Autodesk Inventor part; units mm, degrees
ref_plane "Work Plane1" through (0, 0, 0) normal (0, 0, 1) x (1, 0, 0)
ref_plane "YZ Plane" through (0, 0, 0) normal (1, 0, 0) x (0, 1, 0)
ref_plane "XZ Plane" through (0, 0, 0) normal (0, 1, 0) x (-1, 0, 0)
ref_plane "Work Plane1" through (0, 0, 0) normal (0, 0, 1) x (1, 0, 0)
sketch "Sketch1" plane through (0, 0, 0) normal (0, 0, 1) x (1, 0, 0)
  circle A0 centre (0, 0) radius 21
  circle A1 centre (23.57, -23.57) radius 2
  circle A2 centre (23.57, 23.57) radius 2
  circle A3 centre (-23.57, -23.57) radius 2.5
  circle A4 centre (-23.57, 23.57) radius 2
  circle A5 centre (-23.57, -23.57) radius 2
  circle A6 centre (0, 0) radius 19
  circle A7 centre (-23.57, 23.57) radius 2.5
  circle A8 centre (-23.57, -23.57) radius 2.5
  arc A9 (-29.95, -24.95) -> (-24.95, -29.95) centre (-24.95, -24.95) ccw
  line L0 (24.95, -29.95) -> (-24.95, -29.95)
  arc A10 (24.95, -29.95) -> (29.95, -24.95) centre (24.95, -24.95) ccw
  line L1 (29.95, 24.95) -> (29.95, -24.95)
  arc A11 (29.95, 24.95) -> (24.95, 29.95) centre (24.95, 24.95) ccw
  line L2 (-24.95, 29.95) -> (24.95, 29.95)
  arc A12 (-24.95, 29.95) -> (-29.95, 24.95) centre (-24.95, 24.95) ccw
  line L3 (-29.95, -24.95) -> (-29.95, 24.95)
  circle A13 centre (23.57, -23.57) radius 2.5
  circle A14 centre (23.57, 23.57) radius 2.5
  line L4 (-49.95, -90) -> (-49.95, 90)
  line L5 (-59.95, -90) -> (-49.95, -90)
  line L6 (-59.95, 90) -> (-49.95, 90)
  line L7 (40.2846, 0) -> (-40.2846, 0)
  line L8 (-49.95, -90) -> (-49.95, 90)
  line L9 (-59.95, -90) -> (-49.95, -90)
  line L10 (-49.95, 35.5095) -> (-26.95, 35.5095)
  line L11 (-24.95, 29.95) -> (-49.95, 29.95)
  line L12 (-24.95, -29.95) -> (-49.95, -29.95)
  circle A15 centre (0, 0) radius 22
  line L13 (-32.95, 22) -> (-32.95, -22)
  line L14 (-30.95, -14.95) -> (-49.95, -14.95)
  line L15 (-30.95, 14.95) -> (-49.95, 14.95)
  line L16 (-30.95, -14.95) -> (-30.95, 14.95)
  line L17 (24.7214, -34.026) -> (0, -42.0585)
  line L18 (0, -42.0585) -> (-24.7214, -34.026)
  line L19 (-24.7214, -34.026) -> (-40, -12.9968)
  line L20 (-40, -12.9968) -> (-40, 12.9968)
  line L21 (-40, 12.9968) -> (-24.7214, 34.026)
  line L22 (-24.7214, 34.026) -> (0, 42.0585)
  line L23 (0, 42.0585) -> (24.7214, 34.026)
  line L24 (24.7214, 34.026) -> (40, 12.9968)
  line L25 (40, 12.9968) -> (40, -12.9968)
  line L26 (40, -12.9968) -> (24.7214, -34.026)
  line L27 (-24.7214, -34.026) -> (-49.95, -34.026)
  line L28 (-24.7214, 34.026) -> (-49.95, 34.026)
  arc A16 (-24.7214, -34.026) -> (-24.7214, 34.026) centre (0, 0) ccw
  line L29 (-24.7214, 34.026) -> (-27.8, 34.026)
  line L30 (-27.8, 34.026) -> (-27.8, 80.5095)
  line L31 (-27.8, 80.5095) -> (-49.95, 80.5095)
  line L32 (-49.95, 80.5095) -> (-49.95, 14.95)
  line L33 (-49.95, 14.95) -> (-35.95, 14.95)
  arc A17 (-30.95, 9.95) -> (-35.95, 14.95) centre (-35.95, 9.95) ccw
  line L34 (-30.95, 9.95) -> (-30.95, -9.95)
  arc A18 (-35.95, -14.95) -> (-30.95, -9.95) centre (-35.95, -9.95) ccw
  line L35 (-35.95, -14.95) -> (-49.95, -14.95)
  line L36 (-49.95, -14.95) -> (-49.95, -34.026)
  line L37 (-49.95, -34.026) -> (-24.7214, -34.026)
  circle A19 centre (15.9909, -0.539) radius 1.6
  circle A20 centre (-11.6884, -10.9261) radius 2
  circle A21 centre (11.6884, 10.9261) radius 2
  circle A22 centre (10.9261, -11.6884) radius 2
  circle A23 centre (-15.9909, 0.539) radius 1.6
  circle A24 centre (-0.539, -15.9909) radius 1.6
  circle A25 centre (0, 0) radius 12.5
  circle A26 centre (0.539, 15.9909) radius 1.6
  circle A27 centre (-10.9261, 11.6884) radius 2
  point P0 (0, 0)
  point P1 (-23.2856, -45.1645)
  point P2 (-49.95, -75.9684)
  point P3 (-23.2856, 45.1645)
  point P4 (-49.95, -14.95)
  point P5 (-32.95, 13.95)
  point P6 (-32.95, 14.95)
  dimension "d9" = 1
  dimension "d10" = 15
  dimension "d11" = 15
  dimension "d12" = 1
  dimension "d13" = 40
extrude "Extrusion1" add sketch "Sketch1" along normal blind 10 contours L7 A15 A0 | A0 L7 A15 | A15 L7 L3 A12 L2 A11 L1 | L7 L1 A10 L0 A9 L3 A15 | L7 L25 L26 L17 L18 L19 L12 L0 A10 L1 | L1 A11 L2 L11 L21 L22 L23 L24 L25 L7 | L7 L16 L15 L21 L11 A12 L3 | L3 A9 L12 L19 L14 L16 L7 | L25 A16 | L16 A18 L13 L7 | L7 L13 A17 L16 | L24 A16 | A16 L26 | L13 A18 L14 L19 L20 L7 | L7 L20 L21 L15 A17 L13 | L16 L14 L13 A18 | A17 L13 L15 L16 | L23 A16 | A16 L17 | L19 L27 L4 L12 | L12 L4 L14 L19 | L21 L15 L4 L11 | L11 L4 L28 L21 | L20 L19 L14 L4 L15 L21 | A17 L15 L13 | L13 L14 A18 | L22 A16 | A16 L18 | A1 | A2 | A3 | A4 | A5 | A7 | A13 | A14
sketch "Sketch2" plane through (-49.95, -34.026, 0) normal (-1, 0, 0) x (0, 0, 1)
  line L0 (0, 68.0521) -> (0, 0)
  line L1 (0, 0) -> (10, 0)
  line L2 (10, 68.0521) -> (10, 0)
  line L3 (0, 68.0521) -> (0, 0)
  line L4 (10, 68.0521) -> (10, 0)
  line L5 (0, 68.0521) -> (10, 68.0521)
  line L6 (0, 0) -> (10, 0)
  line L7 (0, 68.0521) -> (10, 68.0521)
  point P0 (0, 34.026)
  point P1 (5, 7.5)
  point P2 (5, 60.5521)
  point P3 (5, 68.0521)
  point P4 (5, 19.076)
  dimension "d24" = 7.5
  dimension "d25" = 7.5
hole "Hole1" at (-49.95, 26.526, 5) at (-49.95, -26.526, 5) direction (1, 0, 0) diameter 3.242 depth 15 tip angle 118
sketch "Sketch3" plane through (0, 0, 10) normal (0, 0, 1) x (1, 0, 0)
  arc A0 (-24.7214, -34.026) -> (-24.7214, 34.026) centre (0, 0) ccw
  line L0 (-24.7214, 34.026) -> (-27.8, 34.026)
  line L1 (-27.8, 34.026) -> (-27.8, 80.5095)
  line L2 (-27.8, 80.5095) -> (-49.95, 80.5095)
  line L3 (-49.95, 80.5095) -> (-49.95, 14.95)
  line L4 (-49.95, 14.95) -> (-35.95, 14.95)
  arc A1 (-30.95, 9.95) -> (-35.95, 14.95) centre (-35.95, 9.95) ccw
  line L5 (-30.95, 9.95) -> (-30.95, -9.95)
  arc A2 (-35.95, -14.95) -> (-30.95, -9.95) centre (-35.95, -9.95) ccw
  line L6 (-35.95, -14.95) -> (-49.95, -14.95)
  line L7 (-49.95, -14.95) -> (-49.95, -34.026)
  line L8 (-49.95, -34.026) -> (-24.7214, -34.026)
  circle A3 centre (15.9909, -0.539) radius 1.6
  circle A4 centre (-11.6884, -10.9261) radius 2
  circle A5 centre (11.6884, 10.9261) radius 2
  circle A6 centre (10.9261, -11.6884) radius 2
  circle A7 centre (-15.9909, 0.539) radius 1.6
  circle A8 centre (-0.539, -15.9909) radius 1.6
  circle A9 centre (0, 0) radius 12.5
  circle A10 centre (0.539, 15.9909) radius 1.6
  circle A11 centre (-10.9261, 11.6884) radius 2
  circle A12 centre (0, 0) radius 19
  circle A13 centre (-23.57, 23.57) radius 2.5
  circle A14 centre (-23.57, -23.57) radius 2.5
  arc A15 (-29.95, -24.95) -> (-24.95, -29.95) centre (-24.95, -24.95) ccw
  line L9 (24.95, -29.95) -> (-24.95, -29.95)
  arc A16 (24.95, -29.95) -> (29.95, -24.95) centre (24.95, -24.95) ccw
  line L10 (29.95, 24.95) -> (29.95, -24.95)
  arc A17 (29.95, 24.95) -> (24.95, 29.95) centre (24.95, 24.95) ccw
  line L11 (-24.95, 29.95) -> (24.95, 29.95)
  arc A18 (-24.95, 29.95) -> (-29.95, 24.95) centre (-24.95, 24.95) ccw
  line L12 (-29.95, -24.95) -> (-29.95, 24.95)
  circle A19 centre (23.57, -23.57) radius 2.5
  circle A20 centre (23.57, 23.57) radius 2.5
  arc A21 (-37.4079, -14.95) -> (-37.4079, 14.95) centre (0, 0) ccw
  line L13 (-27.8, 34.026) -> (-27.8, 29.155)
  line L14 (-49.95, -34.026) -> (-21.5657, -34.026)
  line L15 (-49.95, -34.026) -> (-24.7214, -34.026)
  point P0 (0, 0)
  point P1 (-24.7214, -34.026)
extrude "Extrusion2" cut sketch "Sketch3" against normal blind 10 contours L14 A21 L13 L0 A0
sketch "Sketch4" plane through (0, 0, 10) normal (0, 0, 1) x (1, 0, 0)
  arc A0 (-24.7214, -34.026) -> (-24.7214, 34.026) centre (0, 0) ccw
  line L0 (-24.7214, 34.026) -> (-27.8, 34.026)
  line L1 (-27.8, 34.026) -> (-27.8, 80.5095)
  line L2 (-27.8, 80.5095) -> (-49.95, 80.5095)
  line L3 (-49.95, 80.5095) -> (-49.95, 14.95)
  line L4 (-49.95, 14.95) -> (-35.95, 14.95)
  arc A1 (-30.95, 9.95) -> (-35.95, 14.95) centre (-35.95, 9.95) ccw
  line L5 (-30.95, 9.95) -> (-30.95, -9.95)
  arc A2 (-35.95, -14.95) -> (-30.95, -9.95) centre (-35.95, -9.95) ccw
  line L6 (-35.95, -14.95) -> (-49.95, -14.95)
  line L7 (-49.95, -14.95) -> (-49.95, -34.026)
  line L8 (-49.95, -34.026) -> (-24.7214, -34.026)
  circle A3 centre (15.9909, -0.539) radius 1.6
  circle A4 centre (-11.6884, -10.9261) radius 2
  circle A5 centre (11.6884, 10.9261) radius 2
  circle A6 centre (10.9261, -11.6884) radius 2
  circle A7 centre (-15.9909, 0.539) radius 1.6
  circle A8 centre (-0.539, -15.9909) radius 1.6
  circle A9 centre (0, 0) radius 12.5
  circle A10 centre (0.539, 15.9909) radius 1.6
  circle A11 centre (-10.9261, 11.6884) radius 2
  line L9 (-49.95, -90) -> (-49.95, 90)
  line L10 (-59.95, 90) -> (-49.95, 90)
  line L11 (-49.95, -90) -> (-49.95, 90)
  line L12 (-27.8, 29.155) -> (-27.8, 34.026)
  line L13 (-27.8, 34.026) -> (-49.95, 34.026)
  line L14 (-49.95, 34.026) -> (-49.95, -34.026)
  line L15 (-49.95, -34.026) -> (-21.5657, -34.026)
  arc A12 (-21.5657, -34.026) -> (-27.8, 29.155) centre (0, 0) ccw
  circle A13 centre (0, 0) radius 21
  point P0 (0, 0)
extrude "Extrusion3" add sketch "Sketch4" against normal blind 10 contours L13 L3 L2 L1
fillet "Fillet1" radius 2 2 edges at (-27.8, 29.155, 5) (-21.5657, -34.026, 5)
fillet "Fillet2" radius 1 1 edges at (-27.8, 80.5095, 5)
sketch "Sketch5" plane through (-27.8, 33.5015, 10) normal (1, 0, 0) x (0, 0, -1)
  arc A0 (8, 9.19) -> (10, 11.19) centre (8, 11.19) ccw
  line L0 (10, 49.19) -> (10, 11.19)
  arc A1 (10, 49.19) -> (8, 51.19) centre (8, 49.19) ccw
  line L1 (-60.5, 51.19) -> (8, 51.19)
  arc A2 (-60.5, 51.19) -> (-62.5, 49.19) centre (-60.5, 49.19) ccw
  line L2 (-62.5, 11.19) -> (-62.5, 49.19)
  arc A3 (-62.5, 11.19) -> (-60.5, 9.19) centre (-60.5, 11.19) ccw
  line L3 (8, 9.19) -> (-60.5, 9.19)
  circle A4 centre (-26.25, 30.19) radius 12.6
  circle A5 centre (-26.25, 14.19) radius 2
  arc A6 (-59.6, 14.79) -> (-55.4, 14.79) centre (-57.5, 14.79) ccw
  line L4 (-59.6, 45.59) -> (-59.6, 14.79)
  arc A7 (-55.4, 45.59) -> (-59.6, 45.59) centre (-57.5, 45.59) ccw
  line L5 (-55.4, 14.79) -> (-55.4, 45.59)
  circle A8 centre (-42.25, 30.19) radius 2
  circle A9 centre (-37.5637, 18.8763) radius 1.5
  circle A10 centre (-37.5637, 41.5037) radius 1.5
  circle A11 centre (-14.9363, 18.8763) radius 1.5
  arc A12 (7.1, 45.59) -> (2.9, 45.59) centre (5, 45.59) ccw
  line L6 (7.1, 14.79) -> (7.1, 45.59)
  arc A13 (2.9, 14.79) -> (7.1, 14.79) centre (5, 14.79) ccw
  line L7 (2.9, 45.59) -> (2.9, 14.79)
  circle A14 centre (-10.25, 30.19) radius 2
  circle A15 centre (-14.9363, 41.5037) radius 1.5
  circle A16 centre (-26.25, 46.19) radius 2
  circle A17 centre (-57.5, 11.46) radius 1.621
  circle A18 centre (-57.5, 26.86) radius 1.621
  arc A19 (8, 9.19) -> (10, 11.19) centre (8, 11.19) ccw
  line L8 (10, 49.19) -> (10, 11.19)
  arc A20 (10, 49.19) -> (8, 51.19) centre (8, 49.19) ccw
  line L9 (-60.5, 51.19) -> (8, 51.19)
  arc A21 (-60.5, 51.19) -> (-62.5, 49.19) centre (-60.5, 49.19) ccw
  line L10 (-62.5, 11.19) -> (-62.5, 49.19)
  arc A22 (-62.5, 11.19) -> (-60.5, 9.19) centre (-60.5, 11.19) ccw
  line L11 (8, 9.19) -> (-60.5, 9.19)
  circle A23 centre (-26.25, 30.19) radius 12.6
  circle A24 centre (-26.25, 14.19) radius 2
  arc A25 (-59.6, 14.79) -> (-55.4, 14.79) centre (-57.5, 14.79) ccw
  line L12 (-59.6, 45.59) -> (-59.6, 14.79)
  arc A26 (-55.4, 45.59) -> (-59.6, 45.59) centre (-57.5, 45.59) ccw
  line L13 (-55.4, 14.79) -> (-55.4, 45.59)
  circle A27 centre (-42.25, 30.19) radius 2
  circle A28 centre (-37.5637, 18.8763) radius 1.5
  circle A29 centre (-37.5637, 41.5037) radius 1.5
  circle A30 centre (-14.9363, 18.8763) radius 1.5
  arc A31 (7.1, 45.59) -> (2.9, 45.59) centre (5, 45.59) ccw
  line L14 (7.1, 14.79) -> (7.1, 45.59)
  arc A32 (2.9, 14.79) -> (7.1, 14.79) centre (5, 14.79) ccw
  line L15 (2.9, 45.59) -> (2.9, 14.79)
  circle A33 centre (-10.25, 30.19) radius 2
  circle A34 centre (-14.9363, 41.5037) radius 1.5
  circle A35 centre (-26.25, 46.19) radius 2
  arc A36 (8, 9.19) -> (10, 11.19) centre (8, 11.19) ccw
  line L16 (10, 49.19) -> (10, 11.19)
  arc A37 (10, 49.19) -> (8, 51.19) centre (8, 49.19) ccw
  line L17 (-60.5, 51.19) -> (8, 51.19)
  arc A38 (-60.5, 51.19) -> (-62.5, 49.19) centre (-60.5, 49.19) ccw
  line L18 (-62.5, 11.19) -> (-62.5, 49.19)
  arc A39 (-62.5, 11.19) -> (-60.5, 9.19) centre (-60.5, 11.19) ccw
  line L19 (8, 9.19) -> (-60.5, 9.19)
  circle A40 centre (-26.25, 30.19) radius 12.6
  circle A41 centre (-26.25, 14.19) radius 2
  arc A42 (-59.6, 14.79) -> (-55.4, 14.79) centre (-57.5, 14.79) ccw
  line L20 (-59.6, 45.59) -> (-59.6, 14.79)
  arc A43 (-55.4, 45.59) -> (-59.6, 45.59) centre (-57.5, 45.59) ccw
  line L21 (-55.4, 14.79) -> (-55.4, 45.59)
  circle A44 centre (-42.25, 30.19) radius 2
  circle A45 centre (-37.5637, 18.8763) radius 1.5
  circle A46 centre (-37.5637, 41.5037) radius 1.5
  circle A47 centre (-14.9363, 18.8763) radius 1.5
  arc A48 (7.1, 45.59) -> (2.9, 45.59) centre (5, 45.59) ccw
  line L22 (7.1, 14.79) -> (7.1, 45.59)
  arc A49 (2.9, 14.79) -> (7.1, 14.79) centre (5, 14.79) ccw
  line L23 (2.9, 45.59) -> (2.9, 14.79)
  circle A50 centre (-10.25, 30.19) radius 2
  circle A51 centre (-14.9363, 41.5037) radius 1.5
  circle A52 centre (-26.25, 46.19) radius 2
  point P0 (10, -33.5015)
  point P1 (5, 22.29)
  point P2 (5, 38.09)
  dimension "d47" = 7.5
  dimension "d48" = 7.5
hole "Hole2" at (-27.8, 55.7915, 5) at (-27.8, 71.5915, 5) direction (-1, 0, 0) diameter 3.242 depth 22.15
sketch "Sketch7" plane through (0, 0, 10) normal (0, 0, 1) x (1, 0, 0)
  circle A0 centre (0, 0) radius 32.55
  dimension "d49" = 65.1
extrude "Extrusion5" cut sketch "Sketch7" against normal blind 7
sketch "Sketch10" plane through (0, 0, 0) normal (0, 0, -1) x (-1, 0, 0)
  point P0 (0, 0)
  point P1 (-23.57, -23.57)
  point P2 (-23.57, 23.57)
  point P3 (23.57, 23.57)
  point P4 (23.57, -23.57)
hole "Hole3" at (23.57, -23.57, 0) at (23.57, 23.57, 0) at (-23.57, 23.57, 0) at (-23.57, -23.57, 0) direction (0, 0, 1) diameter 3.242 depth 12 tip angle 118
equation "\"d11\" = d10"
properties part number "motorFrame" material "Aluminum 6061"
CAD build for the part. Positions are in the model's coordinates, mm. A direction names the side the tool comes from. Round coordinates to 2 decimals unless told otherwise and drop trailing zeros. Order: outer loops, then holes, each group sorted by start corner. A loop starts at its lowest first (then second) coordinate and runs counter-clockwise, first axis right, second up. Notation, with made-up numbers: M 75.5,86 L 97.5,86 A16 cw 97.5,101 Z; hole C -4.5,-30.5 d9. An arc over 180 degrees is marked long. Use one line per item in the form item = value.
Q1. Saw through at A-A on x = 0. Give the cut face in (y, z).
Recorded:
outline = M -40.28,0 L -21,0 L -21,3 L -32.55,3 L -32.55,10 L -40.28,10 Z; M 21,0 L 40.28,0 L 40.28,10 L 32.55,10 L 32.55,3 L 21,3 Z
Q2. Probe L1, parallel to Y at x = -43, z = 5 (1 decimal); L2, parallel to Y at x = -33, z = 5; L3, parallel to Y at x = 25, z = 2.25. List the from-to ranges inside material, lowest first.
Recorded:
L1 = -34 to -28.1, -24.9 to 24.9, 28.1 to 54.2, 57.4 to 70, 73.2 to 80.5
L2 = -34.03 to 54.17, 57.41 to 69.97, 73.21 to 80.51
L3 = -31.59 to -24.33, -22.81 to 22.81, 24.33 to 31.59
Q3. Which spindle directions (+Z, -Z, +X, -X, +Y, -Y) get a long thin tool onto all of the face, cutting with end or side? Do faces 5 (the cylindrical face through (0.34, 32.55, 6.55)), 6 (the flat face through (-27.8, 56, 7)), 7 (the flat face through (-36, -34.026, 5)). Say none if no direction does.
Recorded:
face_5 = +Z
face_6 = +Z, -Z, +Y
face_7 = +Z, -Z, -X, -Y
Q4. Saw through at D-D on x = 28. Give the cut face in (y, z), then the cut area to 3 significant figures.
Recorded:
outline = M -28.96,0 L 28.96,0 L 28.96,10 L 16.6,10 L 16.6,3 L -16.6,3 L -16.6,10 L -28.96,10 Z
area = 347 mm^2
Q5. Two-plate mould, pull along Z, no slides. Class faces 1 (the conical face through (-34.145, 26.251, 4.939)), 2 (the flat face through (-0.5, -21.2, 3)), 3 (the cylindrical face through (-42.345, -27.622, 3.805)), 4 (the cylindrical face through (32.55, -0.34, 6.55)): +Z half, -Z half, draft (parallel to the pull), parting line (faces both ways), or undercut.
Recorded:
face_1 = undercut
face_2 = +Z half
face_3 = undercut
face_4 = draft
Q6. Saw through at C-C on z = 8.75. Give the cut face in (x, y), then the cut area to 3 significant figures.
Recorded:
outline = M -49.95,-34.03 L -22.14,-34.03 A2 cw -21.09,-34.32 A40.28 ccw long -24.58,31.92 A2 cw -27.8,33.5 L -27.8,79.51 A1 ccw -28.8,80.51 L -49.95,80.51 Z; hole M -23.99,-22 A1.62 ccw long -22,-23.99 A32.55 ccw 22,-23.99 A1.62 ccw long 23.99,-22 A32.55 ccw 23.99,22 A1.62 ccw long 22,23.99 A32.55 ccw -22,23.99 A1.62 ccw long -23.99,22 A32.55 ccw Z
area = 3,800 mm^2
Q7. Saw through at B-B on y = 0. Give the cut face in (x, z), then the cut area to 3 significant figures.
Recorded:
outline = M -49.95,0 L -21,0 L -21,3 L -32.55,3 L -32.55,10 L -49.95,10 Z; M 21,0 L 40.28,0 L 40.28,10 L 32.55,10 L 32.55,3 L 21,3 Z
area = 321 mm^2
Q8. Flat gauge pins, fed straight in: P1, Ø3.5, axis at x = 23.57, y = 23.57, coming from the +Z side; P2, Ø1.5, axis at x = -15, z = 9, coming from the -Y side; P3, Ø4, axis at y = 55.79, z = 5, coming from the +X side; P4, Ø1, axis at x = -7, z = 2, coming from the +Y side. Where does each tip first touch, or does it go through?
Recorded:
P1 = 10
P2 = -37.68
P3 = -27.8
P4 = 39.76
